```python
from build123d import *

# Parameters (mm, degrees)
SKETCH_2_R          = 6
SKETCH_2_R_2        = 2.6
EXTRUDE_1_DEPTH     = 3
SKETCH_3_R          = 1.8
EXTRUDE_2_DEPTH     = 3
EXTRUDE_3_DEPTH     = 3
EXTRUDE_4_DEPTH     = 3
CHAMFER_2_SIZE      = 1
CUT_EXTRUDE_1_DEPTH = 5


with BuildPart() as part:
    # 草图2 → 凸台-拉伸1 (new body)
    with BuildSketch(Plane(origin=(0, 0, 0), x_dir=(1, 0, 0), z_dir=(0, 1, 0))):
        Circle(SKETCH_2_R)
        Circle(SKETCH_2_R_2, mode=Mode.SUBTRACT)
    extrude(amount=EXTRUDE_1_DEPTH)

    # 草图3 → 凸台-拉伸2 (add)
    with BuildSketch(Plane(origin=(0, 3, 0), x_dir=(1, 0, 0), z_dir=(0, 1, 0))):
        with BuildLine():
            Line((-2.75, 14.603353962), (-2.75, 5.332682252))
            Line((-2.75, 5.332682252), (2.75, 5.332682252))
            Line((2.75, 5.332682252), (2.75, 14.603353962))
            ThreePointArc((2.75, 14.603353962), (0, 17.353353962), (-2.75, 14.603353962))
        make_face()
        with Locations((0, 14.603353962)):
            Circle(SKETCH_3_R, mode=Mode.SUBTRACT)
    extrude(amount=-EXTRUDE_2_DEPTH)

    # 草图5 → 凸台-拉伸3 (add)
    with BuildSketch(Plane(origin=(0, 3, 0), x_dir=(1, 0, 0), z_dir=(0, 1, 0))):
        with BuildLine():
            Line((3.25, 12.603353962), (2.458972536, 11.008619055))
            ThreePointArc((2.458972536, 11.008619055), (6.451860062, 15.228635349), (5, 9.603353962))
            Line((5, 9.603353962), (5, 10.853353962))
            ThreePointArc((5, 10.853353962), (6.237436867, 13.840790829), (3.25, 12.603353962))
        make_face()
    extrude(amount=-EXTRUDE_3_DEPTH)

    # 草图6 → 凸台-拉伸4 (add)
    with BuildSketch(Plane(origin=(0, 3, 0), x_dir=(1, 0, 0), z_dir=(0, 1, 0))):
        Polygon((5.032823561, -3.266601752), (40.031302406, -22.854160513), (36.087762843, -11.678430785), (36.087762843, -4.064639853), (40.031302406, 1.52127196), (40.031302406, 5.037888577), (45.031302406, 5.037888577), (45.031302406, 8.037888577), (40.031302406, 8.037888577), (29.357105905, 1.733398248), (5.032823561, 1.733398248), align=None)
    extrude(amount=-EXTRUDE_4_DEPTH)

    # 倒角2
    chamfer_2_edges = [part.edges().sort_by_distance(p)[0] for p in [
        (45.031302406, 1.5, -8.037888577),
    ]]
    chamfer(chamfer_2_edges, length=CHAMFER_2_SIZE)

    # 草图7 → 切除-拉伸1 (cut, symmetric)
    with BuildSketch(Plane(origin=(0, 3, 0), x_dir=(1, 0, 0), z_dir=(0, 1, 0))):
        Polygon((11.673818528, -3.545473406), (24.087762843, -10.49317147), (24.087762843, -1.266601752), (11.673818528, -1.266601752), align=None)
    extrude(amount=CUT_EXTRUDE_1_DEPTH, both=True, mode=Mode.SUBTRACT)


solid = part.part
```
Can you work these out from the model? Positions are in its coordinate system, mm. A direction names the side the tool comes from. Give positions to 0.01 mm unless a question says otherwise; leave off trailing zeros. Write each loop counter-clockwise with the first axis right and the second up, starting at its lowest first coordinate (ties: lowest second). Pieces come first, ordered by that corner, then holes. Notation, with made-up numbers: (63.25, 35) - (82.25, 35) arc R18 cw to (82.25, 63) - close; hole circle Ø1 at (1.5, -28). An arc over 180 degrees is marked (long way). Write item = value, one per line. Start each with the question number.
1. Imagine slicing it at A-A (x = 0). Please give me the cut outline in (y, z).
2. Thinking about a two-plate mould opening in Z: for faces 6 (the face through (42, 2, -5.038)), 7 (the face through (4.634, 1.479, -3.811)), 8 (the face through (45.031, 2, -6)), which applies, released by +Z, released by -Z, zero draft, split by the parting line, or undercut?
3. Imagine slicing it at D-D (x = 22.5). Please give me the cut outline in (y, z).
4. On a 3-axis mill with a long thin cutter (end or side, diameter ignored), from which of +Z, -Z, +X, -X, +Y, -Y can I reach the whole of each face in a straight line? I mean faces 1 (the face through (18, 0, 1)), 2 (the face through (36.088, 2, 8)), 3 (the face through (44.54, 1.52, -7.53)), 4 (the face through (17.79, 1.52, 6.97)), 5 (the face through (34.77, 1.52, -4.93)). Say none if no direction works.
5. Imagine slicing it at C-C (z = 0). Please give me the cut outline in (x, y).
6. For pin 1 (1.5 mm diameter, centred on x = 28.5, y = 2.5, fed in from +Z); pin 2 (6 mm diameter, centred on x = 0, z = 0, fed in from -Y); pin 3 (1 mm diameter, centred on y = 2, z = 1, fed in from -X); pin 4 (1.5 mm diameter, centred on x = 42.5, y = 2, fed in from -Z), each with a flat end and sliding along its axis, tell me the tip position at first contact or that it passes through.
7. Please list where these lines run through material, in increasing order: line 1 (Z direction, x = 0, y = 0.9); line 2 (Z direction, x = 1.5, y = 1.1); line 3 (X direction, y = 1.65, z = 5.5).
8. Imagine slicing it at B-B (y = 2.5). Count the separate pieces of the cut face and the enclosed holes in it, and give its area (3 significant figures).
Worked answers:
q1.outline = (0, -17.35) - (3, -17.35) - (3, -16.4) - (0, -16.4) - close; (0, -12.8) - (3, -12.8) - (3, -2.6) - (0, -2.6) - close; (0, 2.6) - (3, 2.6) - (3, 6) - (0, 6) - close
q2.face_6 = released by +Z
q2.face_7 = undercut
q2.face_8 = zero draft
q3.outline = (0, -1.73) - (3, -1.73) - (3, 1.27) - (0, 1.27) - close; (0, 9.6) - (3, 9.6) - (3, 13.04) - (0, 13.04) - close
q4.face_1 = +Z, -Z, +X, -X, -Y
q4.face_2 = +X, +Y, -Y
q4.face_3 = -Z, +X, +Y, -Y
q4.face_4 = +Y, -Y
q4.face_5 = -Z, +Y, -Y
q5.outline = (-6, 0) - (-2.6, 0) - (-2.6, 3) - (-6, 3) - close; (2.6, 0) - (38.96, 0) - (38.96, 3) - (2.6, 3) - close
q6.pin_1 = 16.82
q6.pin_2 = 0
q6.pin_3 = -5.98
q6.pin_4 = -8.04
q7.line_1 = -17.35 to -16.4, -12.8 to -2.6, 2.6 to 6
q7.line_2 = -16.91 to -15.6, -13.61 to -2.12, 2.12 to 5.81
q7.line_3 = -2.4 to 2.4, 9.02 to 15.17, 24.09 to 36.09
q8.separate_pieces = 1
q8.enclosed_holes = 3
q8.area = 583 mm2
